```python
from build123d import *

# Parameters (mm, degrees)
BASENUT_DEPTH = 16
GRVSKE_W      = 6
GRVSKE_H      = 2.75
DOMEFILLET_R  = 1


with BuildPart() as part:
    # BaseNutSke → BaseNut (new body)
    with BuildSketch(Plane(origin=(0, 0, 0), x_dir=(0, 0, -1), z_dir=(1, 0, 0))):
        Polygon((15, 8.660254038), (15, -8.660254038), (0, -17.320508076), (-15, -8.660254038), (-15, 8.660254038), (0, 17.320508076), align=None)
    extrude(amount=BASENUT_DEPTH)

    # DomeSke → Dome (revolve)
    with BuildSketch(Plane.XY, mode=Mode.PRIVATE) as dome_sk:
        with BuildLine():
            Line((34, 0), (0, 0))
            Line((0, 0), (0, 13.5))
            Line((0, 13.5), (20.5, 13.5))
            ThreePointArc((20.5, 13.5), (30.045941546, 9.545941546), (34, 0))
        make_face()
    revolve(dome_sk.sketch.rotate(Axis((0, 0, 0), (1, 0, 0)), 90), axis=Axis((0, 0, 0), (1, 0, 0)))

    # Sketch4 → DoubleChamfer (revolve, cut)
    with BuildSketch(Plane.XY):
        Polygon((0, 15), (2.783121635, 19.820508076), (13.216878365, 19.820508076), (16, 15), (18, 15), (18, 30), (-2, 30), (-2, 15), align=None)
    revolve(axis=Axis((0, 0, 0), (1, 0, 0)), mode=Mode.SUBTRACT)

    # TapDriSke → TapDrill (revolve, cut)
    with BuildSketch(Plane.XY, mode=Mode.PRIVATE) as tapdrill_sk:
        Polygon((0, 8.75), (27, 8.75), (32.257530416, 0), (0, 0), align=None)
    revolve(tapdrill_sk.sketch.rotate(Axis((0, 0, 0), (1, 0, 0)), 90), axis=Axis((0, 0, 0), (1, 0, 0)), mode=Mode.SUBTRACT)

    # GrvSke → Groove (revolve, cut)
    with BuildSketch(Plane.XY, mode=Mode.PRIVATE) as groove_sk:
        with Locations((19, 9.125)):
            Rectangle(GRVSKE_W, GRVSKE_H)
    revolve(groove_sk.sketch.rotate(Axis((0, 0, 0), (1, 0, 0)), 90), axis=Axis((0, 0, 0), (1, 0, 0)), mode=Mode.SUBTRACT)

    # EndChamferSketch → EndChamfer (revolve, cut)
    with BuildSketch(Plane.XY):
        Polygon((-0.0254, 10), (0.0254, 10), (0.988185365, 8.625), (-0.0254, 8.625), align=None)
    revolve(axis=Axis((0, 0, 0), (-1, 0, 0)), mode=Mode.SUBTRACT)

    # DomeFillet
    domefillet_edges = [part.edges().sort_by_distance(p)[0] for p in [
        (16, 0, -13.5),
    ]]
    fillet(domefillet_edges, radius=DOMEFILLET_R)


solid = part.part
```
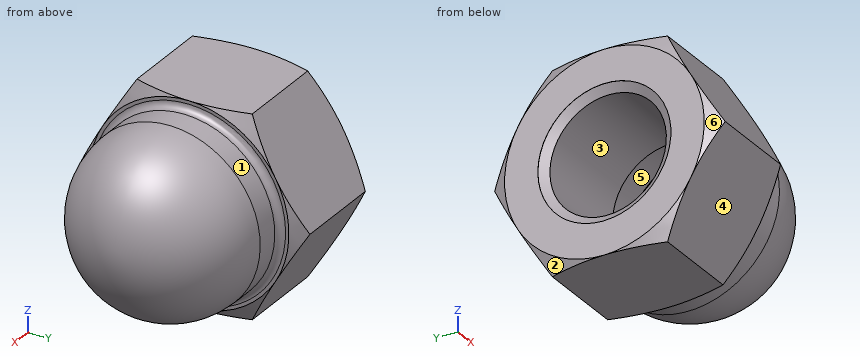
Geometry check sheet. Reference: the model listing, model coordinates, mm. Face numbers are marked on the shaded views. A direction names the side the tool comes from. Give positions to 0.01 mm unless a question says otherwise; leave off trailing zeros. Write each loop counter-clockwise with the first axis right and the second up, starting at its lowest first coordinate (ties: lowest second). Pieces come first, ordered by that corner, then holes. Notation, with made-up numbers: (34.25, -0.75) - (60.25, -0.75) arc R9 cw to (60.25, 5.25) - close; hole circle Ø1 at (34, 14). An arc over 180 degrees is marked (long way). Use a Markdown table: item, result.
Q1. Thickness scan on L1, parallel to Y at x = 19.2, z = 0; L2, parallel to Y at x = 13, z = 0; L3, parallel to X at y = -14, z = -4.5. Record the ranges inside material, lowest first. Write a range as [from, to].
Computed:
| item | result |
|---|---|
| L1 | y = [-13.5, -10.5], [10.5, 13.5] |
| L2 | y = [-17.32, -8.75], [8.75, 17.32] |
| L3 | x = [0, 16] |
Q2. Draft check along X on the marked faces 4, 5 and 6. Enter one of: pulls with the +X half, pulls with the -X half, needs draft (parallel to the pull), parting line crosses it, or undercut.
Computed:
| item | result |
|---|---|
| face 4 | needs draft |
| face 5 | undercut |
| face 6 | pulls with the -X half |
Q3. Set-up check for the marked faces 1, 2 and 3: record each of +Z, -Z, +X, -X, +Y, -Y from which the full face is reachable in a straight line by a thin tool's end or side.
Computed:
| item | result |
|---|---|
| face 1 | +X |
| face 2 | -Z, -X, +Y |
| face 3 | -X |
Q4. Go/stop test with flat-tipped pins: P1, Ø12, axis at x = 3.5, z = 10.5, coming from the +Y side; P2, Ø4, axis at x = 15, z = 2, coming from the -Y side; P3, Ø10, axis at y = 3, z = -10, coming from the +X side; P4, Ø17, axis at y = 2.5, z = -1.5, coming from the -X side. Record where each tip stops, or that it passes through.
Computed:
| item | result |
|---|---|
| P1 | stops at y = 14.72 |
| P2 | stops at y = -17.3 |
| P3 | stops at x = 32.86 |
| P4 | stops at x = 0 |
Q5. Section check A-A, the plane x = 7.5. Enter the section's corners in (y, z), then the cut area to 3 significant figures.
Computed:
| item | result |
|---|---|
| outline | (-17.32, 0) - (-8.66, -15) - (8.66, -15) - (17.32, 0) - (8.66, 15) - (-8.66, 15) - close; hole circle Ø17.5 at (0, 0) |
| area | 539 mm² |
